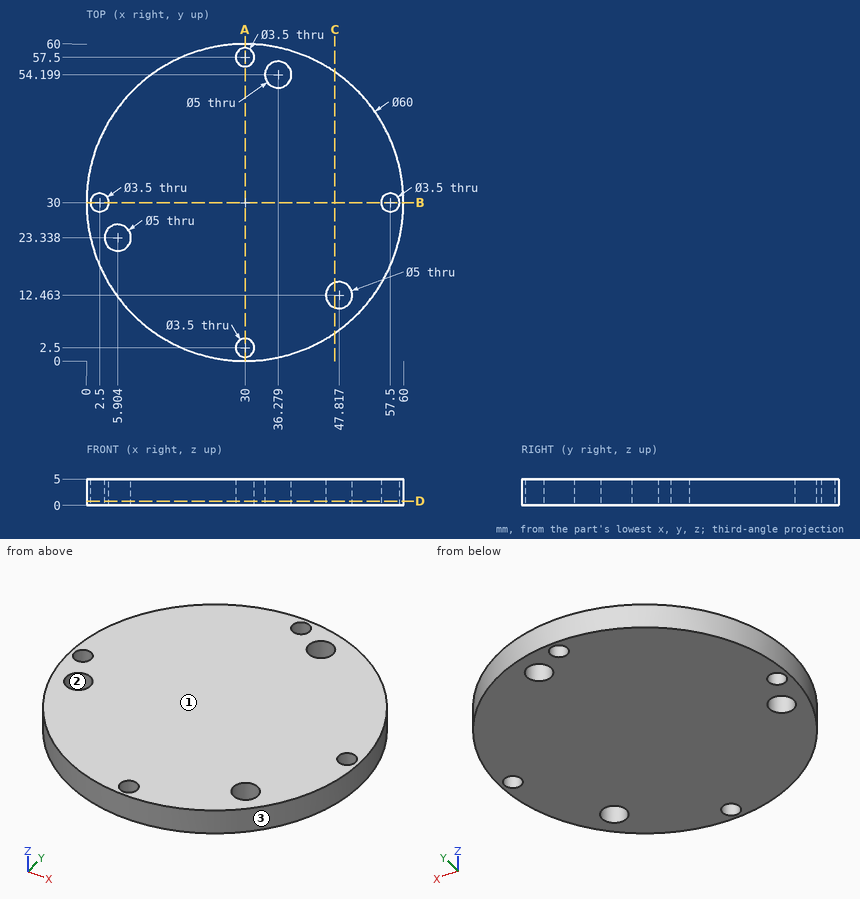
Source: three-view drawing plus pictorial views. Frame: mm from the lowest corner of the part. Round coordinates to 2 decimals unless told otherwise and drop trailing zeros. Order: outer loops, then holes, each group sorted by start corner. A loop starts at its lowest first (then second) coordinate and runs counter-clockwise, first axis right, second up. Notation, with made-up numbers: M 89.5,66 L 94.5,66 A6 cw 94.5,72 Z; hole C -10.75,-9.5 d1. An arc over 180 degrees is marked long. One line per item, written item: value.
(1) Line query: probe 1 along Y at (x, z) = (30, 1.7); probe 2 along X at (y, z) = (24.5, 3.9); probe 3 along Y at (x, z) = (7.5, 2.7) (1 decimal). Output: solid intervals per line, ascending. Write a range as [from, to].
Result sheet:
probe 1: [0, 0.75], [4.25, 55.75], [59.25, 60]
probe 2: [0.51, 3.69], [8.12, 59.49]
probe 3: [10.2, 21.4], [25.3, 49.8]
(2) Cut plane D-D (z = 0.8). Return the cut outline in (x, y).
Result sheet:
outline: C 30,30 d60; hole C 2.5,30 d3.5; hole C 5.9,23.34 d5; hole C 30,2.5 d3.5; hole C 30,57.5 d3.5; hole C 36.28,54.2 d5; hole C 47.82,12.46 d5; hole C 57.5,30 d3.5
(3) Pull-direction query (X, two-part tool) for the marked faces 1, 2 and 3; classes: pulls with the +X half, pulls with the -X half, needs draft (parallel to the pull), parting line crosses it, or undercut.
Result sheet:
face 1: needs draft
face 2: undercut
face 3: parting line crosses it
(4) Pin query (flat end, axial travel): P1, Ø4.5, axis at x = 5.9, y = 23.34, coming from the +Z side; P2, Ø5.5, axis at x = 2.5, y = 30, coming from the -Z side; P3, Ø1.5, axis at y = 34.5, z = 4, coming from the -X side (1 decimal). Return the tip coordinate at first contact, or that it passes through.
Result sheet:
P1: through
P2: z = 0
P3: x = 0.2
(5) Cut plane A-A (x = 30). Return the cut outline in (y, z).
Result sheet:
outline: M 0,0 L 0.75,0 L 0.75,5 L 0,5 Z; M 4.25,0 L 55.75,0 L 55.75,5 L 4.25,5 Z; M 59.25,0 L 60,0 L 60,5 L 59.25,5 Z
(6) Cut plane C-C (x = 47). Return the cut outline in (y, z) (1 decimal).
Result sheet:
outline: M 5.3,0 L 10.1,0 L 10.1,5 L 5.3,5 Z; M 14.8,0 L 54.7,0 L 54.7,5 L 14.8,5 Z
